Check sheet for the modelled part. Datum: model origin and axes. Units: mm. Face numbers are marked on the shaded views. A direction names the side the tool comes from. Coordinates: 2 decimals unless noted, no trailing zeros. Loops run counter-clockwise (first coordinate to the right, second up) from the corner with the lowest first, then second, coordinate; pieces in that order, holes last. Notation, with made-up numbers: (20.25, -6) -> (79.25, -6) arc R8 cw to (79.25, 2) -> close; hole circle Ø8 at (60.25, 73.25). An arc over 180 degrees is marked (long way). Use one line per item in the form item = value.
from build123d import *

# Parameters (mm, degrees)
ESQUISSE1_W             = 36.200001836
ESQUISSE1_H             = 29.499999305
BOSS_EXTRU_1_DEPTH      = 5
ESQUISSE2_W             = 33.052998595
ESQUISSE2_H             = 12.371999211
ENL_V_MAT_EXTRU_1_DEPTH = 5
BOSS_EXTRU_2_START      = 5
ESQUISSE3_W             = 4.558359629
ESQUISSE3_H             = 12.371999211
ESQUISSE3_W_2           = 4.999999888
ESQUISSE3_H_2           = 12.380001135
BOSS_EXTRU_2_DEPTH      = 3.5
BOSS_EXTRU_5_DEPTH      = 2
BOSS_EXTRU_5_DEPTH_BACK = 1
BOSS_EXTRU_5_START      = 6
ESQUISSE4_R             = 12.398139185
ENL_V_MAT_EXTRU_3_REACH = 49.691
ESQUISSE6_W             = 2.256513492
ESQUISSE6_H             = 12.371999211
SKETCH4_R               = 21
SKETCH4_R_2             = 19
BOSS_EXTRUDE2_DEPTH     = 10
SKETCH5_R               = 20
SKETCH5_R_2             = 12.35
BOSS_EXTRUDE7_DEPTH     = 0.75


with BuildPart() as part:
    # Esquisse1 → Boss.-Extru.1 (new body)
    with BuildSketch(Plane.XY):
        with Locations((5.10000065, -15.249999676)):
            Rectangle(ESQUISSE1_W, ESQUISSE1_H)
    extrude(amount=BOSS_EXTRU_1_DEPTH)

    # Esquisse2 → Enlèv. mat.-Extru.1 (cut)
    with BuildSketch(Plane.XY):
        with Locations((4.523499403, -15.158999246)):
            Rectangle(ESQUISSE2_W, ESQUISSE2_H)
    extrude(amount=ENL_V_MAT_EXTRU_1_DEPTH, mode=Mode.SUBTRACT)

    # Esquisse3 → Boss.-Extru.2 (add)
    with BuildSketch(Plane.XY.offset(BOSS_EXTRU_2_START)):
        with Locations((18.770818887, -15.158999246)):
            Rectangle(ESQUISSE3_W, ESQUISSE3_H)
        with Locations((-9.50299995, -15.163000208)):
            Rectangle(ESQUISSE3_W_2, ESQUISSE3_H_2)
    extrude(amount=-BOSS_EXTRU_2_DEPTH)

    # Esquisse4 → Boss.-Extru.5 (add, two sides: drawn at the far end of the back side and taken through both)
    with BuildSketch(Plane.XY.offset(BOSS_EXTRU_5_START - BOSS_EXTRU_5_DEPTH_BACK)):
        with Locations((10.5484362, -15.38812394)):
            Circle(ESQUISSE4_R)
        with BuildLine():
            ThreePointArc((5.299216058, -19.01722353), (16.929328279, -15.482422447), (5.408748548, -11.605494329))
            ThreePointArc((5.408748548, -11.605494329), (0.800592824, -15.244067738), (5.299216058, -19.01722353))
        make_face(mode=Mode.SUBTRACT)
    extrude(amount=BOSS_EXTRU_5_DEPTH + BOSS_EXTRU_5_DEPTH_BACK)

    # Enlèv. mat.-Extru.3: up to this face of the body (flat: up to its plane)
    enl_v_mat_extru_3_end = Plane(part.part.faces().sort_by_distance((16.491639072, -15.158999246, 3.25))[0])
    # Esquisse6 → Enlèv. mat.-Extru.3 (cut, up to the picked face)
    with BuildSketch(Plane.ZY.offset(13.000000268), mode=Mode.PRIVATE) as enl_v_mat_extru_3_sk1:
        with Locations((6.128256634, -15.158999246)):
            Rectangle(ESQUISSE6_W, ESQUISSE6_H)
    enl_v_mat_extru_3_tool1 = split(extrude(enl_v_mat_extru_3_sk1.sketch, amount=-ENL_V_MAT_EXTRU_3_REACH, mode=Mode.PRIVATE), bisect_by=enl_v_mat_extru_3_end, keep=Keep.BOTH, mode=Mode.PRIVATE)
    add(enl_v_mat_extru_3_tool1.solids().sort_by(Axis((-13, -15.158999, 6.128257), (1, 0, 0)))[0], mode=Mode.SUBTRACT)

    # Sketch4 → Boss-Extrude2 (add)
    with BuildSketch(Plane.XY.offset(5)):
        with Locations(Location((10.5484362, -15.38812394, 0), (0, 0, 224.09128758))):
            Circle(SKETCH4_R)
        with Locations(Location((10.5484362, -15.38812394, 0), (0, 0, 230.268304167))):
            Circle(SKETCH4_R_2, mode=Mode.SUBTRACT)
    extrude(amount=BOSS_EXTRUDE2_DEPTH)

    # Sketch5 → Boss-Extrude7 (add)
    with BuildSketch(Plane.XY.offset(8)):
        with Locations((10.5484362, -15.38812394)):
            Circle(SKETCH5_R)
        with Locations((10.5484362, -15.38812394)):
            Circle(SKETCH5_R_2, mode=Mode.SUBTRACT)
    extrude(amount=-BOSS_EXTRUDE7_DEPTH)


solid = part.part
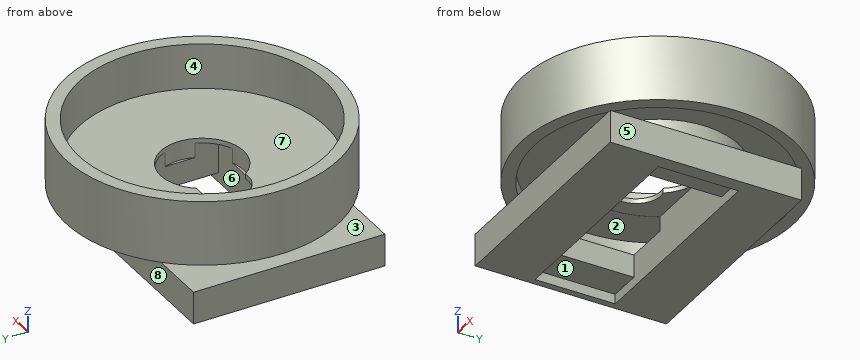
(1) Tool access check on the marked faces 5, 6, 7 and 8. Record the directions out of +Z, -Z, +X, -X, +Y, -Y that give a thin tool (end or side, any length) a straight path to the whole face; none if there is none.
Established:
face_5 = -Z, +X, +Y, -Y
face_6 = -Z
face_7 = +Z
face_8 = -Z, +X, -X, +Y
(2) Mould release check, pull along Z, two halves, no side actions. Record for the marked faces 1, 2, 3 and 4: +Z half, -Z half, draft (parallel to the pull), parting line (faces both ways), or undercut.
Established:
face_1 = -Z half
face_2 = undercut
face_3 = +Z half
face_4 = draft
(3) Scan lines: line 1 along Y through (x, z) = (-0.5, 3) (3 decimals); line 2 along Z through (x, y) = (0.5, -24); line 3 along X through (y, z) = (-15.3, 7.75). Record each from-to range of solid material in increasing order.
Established:
line_1 = -30 to -21.345, -8.973 to -0.5
line_2 = 0 to 5, 7.25 to 8
line_3 = -10.45 to 0.8, 16.93 to 31.55
(4) Section check C-C, the plane y = -4. Record the boundary of the cut face in (x, z).
Established:
outline = (-13, 0) -> (23.2, 0) -> (23.2, 5) -> (15.45, 5) -> (15.45, 7.25) -> (25.76, 7.25) -> (25.76, 5) -> (28.19, 5) -> (28.19, 15) -> (25.76, 15) -> (25.76, 8) -> (-4.66, 8) -> (-4.66, 15) -> (-7.1, 15) -> (-7.1, 5) -> (-13, 5) -> close; hole (-4.66, 5) -> (5.65, 5) -> (5.65, 7.25) -> (-4.66, 7.25) -> close
(5) Go/stop test with flat-tipped pins: P1, Ø4, axis at y = -2, z = 8.5, coming from the -X side; P2, Ø23, axis at x = 10.55, y = -15.39, coming from the +Z side; P3, Ø3, axis at x = -1, z = 8, coming from the -Y side. Record where each tip stops, or that it passes through.
Established:
P1 = -7.1
P2 = 8
P3 = -33.83
(6) Section check A-A, the plane x = 10. Record the boundary of the cut face in (y, z) (3 decimals).
Established:
outline = (-36.381, 5) -> (-34.38, 5) -> (-34.38, 7.25) -> (-27.774, 7.25) -> (-27.774, 5) -> (-30, 5) -> (-30, 0) -> (-21.345, 0) -> (-21.345, 5) -> (-21.746, 5) -> (-21.746, 8) -> (-34.38, 8) -> (-34.38, 15) -> (-36.381, 15) -> close; (-9.03, 7.257) -> (-8.973, 7.257) -> (-8.973, 0) -> (-0.5, 0) -> (-0.5, 5) -> (-3.002, 5) -> (-3.002, 7.25) -> (3.604, 7.25) -> (3.604, 5) -> (5.605, 5) -> (5.605, 15) -> (3.604, 15) -> (3.604, 8) -> (-9.03, 8) -> close
(7) Section check D-D, the plane z = 12.5. Record the boundary of the cut face in (x, y).
Established:
outline = circle Ø42 at (10.55, -15.39); hole circle Ø38 at (10.55, -15.39)
